Job drawing, mm, ordinate dimensions from the low corner. One solid piece. A direction names the side the tool comes from. Give positions to 0.01 mm unless a question says otherwise; leave off trailing zeros. Loops run counter-clockwise (first coordinate to the right, second up) from the corner with the lowest first, then second, coordinate; pieces in that order, holes last. Notation, with made-up numbers: (-24.75, 61.5) - (26.25, 61.5) arc R8 cw to (26.25, 68.5) - close; hole circle Ø8 at (81, 64). An arc over 180 degrees is marked (long way). Use a Markdown table: item, result.
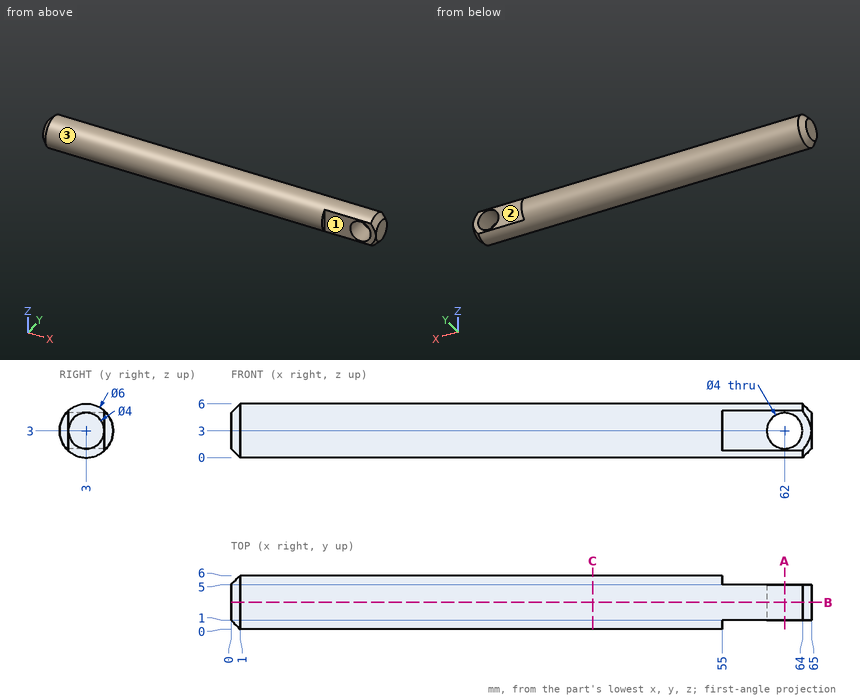
(1) Pin check, flat tips, straight feed: P1, Ø1.5, axis at x = 58, y = 5.5, coming from the +Z side; P2, Ø2, axis at y = 2.5, z = 5, coming from the +X side; P3, Ø2.5, axis at x = 62, z = 3, coming from the +Y side; P4, Ø2, axis at x = 32.5, z = 1, coming from the -Y side. Stop position of each tip, or through.
Computed:
| item | result |
|---|---|
| P1 | z = 5.44 |
| P2 | x = 65 |
| P3 | through |
| P4 | y = 0.17 |
(2) Slice it at A-A, the plane x = 62. Write the cut outline in (y, z).
Computed:
| item | result |
|---|---|
| outline | (1, 0.76) arc R3 ccw to (5, 0.76) - (5, 1) - (1, 1) - close; (1, 5) - (5, 5) - (5, 5.24) arc R3 ccw to (1, 5.24) - close |
(3) 3-axis set-ups, long thin cutter, end or side, ignore diameter. For the marked faces 1, 2 and 3: which of +Z, -Z, +X, -X, +Y, -Y reach the whole face in a straight line?
Computed:
| item | result |
|---|---|
| face 1 | +Z, -Z, +X, -Y |
| face 2 | +Z, -Z, +X, +Y |
| face 3 | +X, -X |
(4) Drill centre lines: probe 1 along X at (y, z) = (4.5, 2.85); probe 2 along Y at (x, z) = (28, 3.2); probe 3 along Z at (x, y) = (62, 3.6). Where is each one in solid material? Low to high. Write a range as [from, to].
Computed:
| item | result |
|---|---|
| probe 1 | [0, 60.01], [63.99, 65] |
| probe 2 | [0.01, 5.99] |
| probe 3 | [0.06, 1], [5, 5.94] |
(5) Slice it at C-C, the plane x = 40.5. Write the cut outline in (y, z), plus the area to 3 significant figures.
Computed:
| item | result |
|---|---|
| outline | circle Ø6 at (3, 3) |
| area | 28.3 mm² |
(6) Slice it at B-B, the plane y = 3. Write the cut outline in (x, z).
Computed:
| item | result |
|---|---|
| outline | (0, 1) - (1, 0) - (64, 0) - (65, 1) - (65, 5) - (64, 6) - (1, 6) - (0, 5) - close; hole circle Ø4 at (62, 3) |
